Geometry check sheet. Reference: drawing and pictorial views, mm from the part's lowest x, y, z. Coordinates: 2 decimals unless noted, no trailing zeros. Loops run counter-clockwise (first coordinate to the right, second up) from the corner with the lowest first, then second, coordinate; pieces in that order, holes last. Notation, with made-up numbers: (-33.75, 61) - (20.25, 61) arc R16 cw to (20.25, 81) - close; hole circle Ø7 at (44.25, 57.5). An arc over 180 degrees is marked (long way). Use a Markdown table: item, result. Add a question column.
1) Go/stop test with flat-tipped pins: P1, Ø1.5, axis at x = 35, z = 10.5, coming from the +Y side; P2, Ø3, axis at x = 9.5, z = 21, coming from the +Y side; P3, Ø3, axis at y = 10, z = 29, coming from the +X side. Record where each tip stops, or that it passes through.
2) Thickness scan on line 1 (Y direction, x = 26.5, z = 7); line 2 (X direction, y = 26, z = 15); line 3 (X direction, y = 28, z = 16). Record the ranges inside material, lowest first.
3) Sectioned sample at A-A, the plane y = 26.5. Enter the section's corners in (x, z), then the cut area to 3 significant figures.
4) Sectioned sample at B-B, the plane z = 29. Enter the section's corners in (x, y), then the cut area to 3 significant figures.
5) Draft check along Y on the marked faces 1, 2 and 3. Enter one of: pulls with the +Y half, pulls with the -Y half, needs draft (parallel to the pull), parting line crosses it, or undercut.
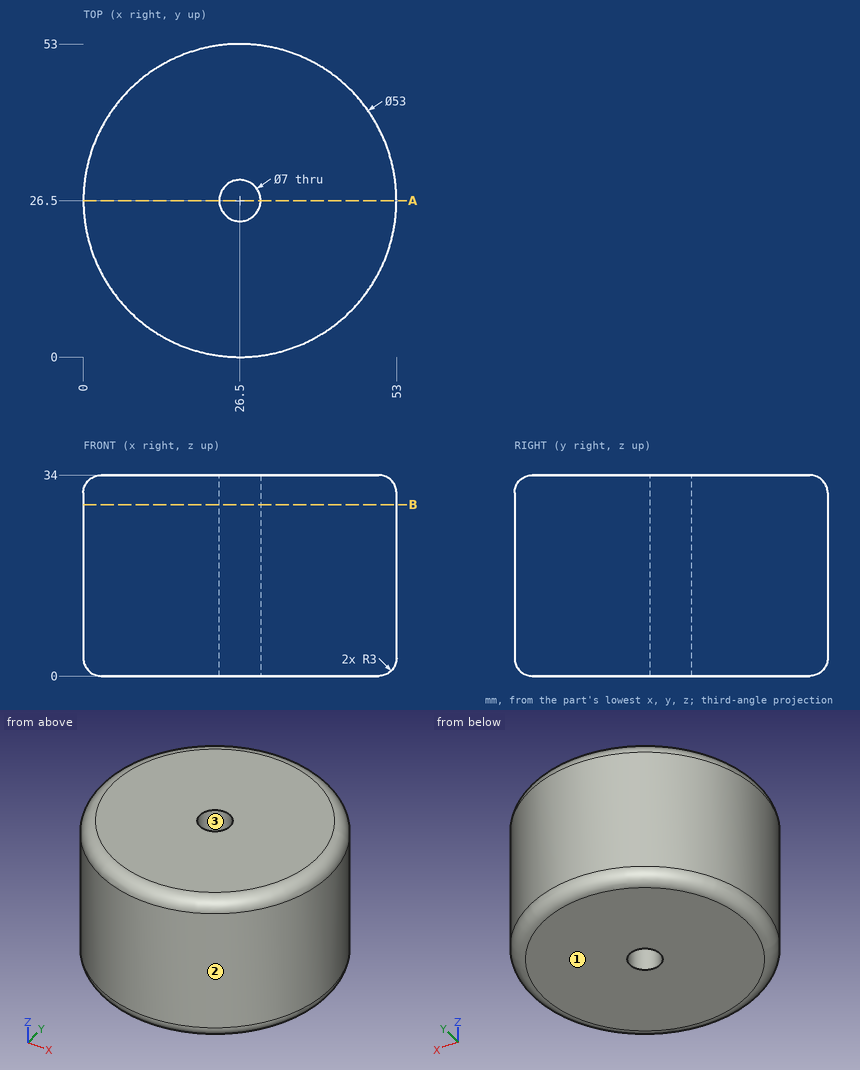
Solved:
| question | item | result |
|---|---|---|
| 1 | P1 | stops at y = 51.84 |
| 1 | P2 | stops at y = 47.99 |
| 1 | P3 | stops at x = 48.35 |
| 2 | line 1 | y = 0 to 23, 30 to 53 |
| 2 | line 2 | x = 0 to 23.04, 29.96 to 53 |
| 2 | line 3 | x = 0.04 to 23.34, 29.66 to 52.96 |
| 3 | outline | (0, 3) arc R3 ccw to (3, 0) - (23, 0) - (23, 34) - (3, 34) arc R3 ccw to (0, 31) - close; (30, 0) - (50, 0) arc R3 ccw to (53, 3) - (53, 31) arc R3 ccw to (50, 34) - (30, 34) - close |
| 3 | area | 1,560 mm2 |
| 4 | outline | circle Ø53 at (26.5, 26.5); hole circle Ø7 at (26.5, 26.5) |
| 4 | area | 2,170 mm2 |
| 5 | face 1 | needs draft |
| 5 | face 2 | parting line crosses it |
| 5 | face 3 | undercut |
